from build123d import *

# Parameters (mm, degrees)
SKETCH1_R           = 8
SKETCH1_R_2         = 8.5
BOSS_EXTRUDE1_DEPTH = 35
BOSS_EXTRUDE3_DEPTH = 12
CUT_EXTRUDE1_DEPTH  = 14.407172
SKETCH7_R           = 8.5
BOSS_EXTRUDE4_DEPTH = 15
SKETCH7_3_R         = 5
CUT_EXTRUDE2_DEPTH  = 15
SKETCH7_4_R         = 6.165
CUT_EXTRUDE3_DEPTH  = 1.5
SKETCH7_5_R         = 1.425
CUT_EXTRUDE4_DEPTH  = 8


with BuildPart() as part:
    # Sketch1 → Boss-Extrude1 (new body)
    with BuildSketch(Plane(origin=(0, 0, 0), x_dir=(1, 0, 0), z_dir=(0, 1, 0))):
        with BuildLine():
            ThreePointArc((-50.982546594, 7.568285795), (-54, 0), (-50.982546594, -7.568285795))
            Line((-50.982546594, -7.568285795), (-54, -11))
            Line((-54, -11), (-54, -25.34082208))
            Line((-54, -25.34082208), (-47.34082208, -32))
            Line((-47.34082208, -32), (5, -32))
            Line((5, -32), (15.759494281, -19.407172386))
            ThreePointArc((15.759494281, -19.407172386), (18.621320344, -18.621320344), (19.407172386, -15.759494281))
            ThreePointArc((19.407172386, -15.759494281), (25, 0), (19.407172386, 15.759494281))
            ThreePointArc((19.407172386, 15.759494281), (18.621320344, 18.621320344), (15.759494281, 19.407172386))
            Line((15.759494281, 19.407172386), (5, 32))
            Line((5, 32), (1, 32))
            Line((1, 32), (1, 21.977260976))
            ThreePointArc((1, 21.977260976), (8.243992543, 20.396974946), (14.551632211, 16.5))
            Line((14.551632211, 16.5), (16.5, 16.5))
            Line((16.5, 16.5), (16.5, 14.551632211))
            ThreePointArc((16.5, 14.551632211), (22, 0), (16.5, -14.551632211))
            Line((16.5, -14.551632211), (16.5, -16.5))
            Line((16.5, -16.5), (14.551632211, -16.5))
            ThreePointArc((14.551632211, -16.5), (0, -22), (-14.551632211, -16.5))
            Line((-14.551632211, -16.5), (-16.5, -16.5))
            Line((-16.5, -16.5), (-16.5, -14.551632211))
            ThreePointArc((-16.5, -14.551632211), (-22, 0), (-16.5, 14.551632211))
            Line((-16.5, 14.551632211), (-16.5, 16.5))
            Line((-16.5, 16.5), (-14.551632211, 16.5))
            ThreePointArc((-14.551632211, 16.5), (-8.243992543, 20.396974946), (-1, 21.977260976))
            Line((-1, 21.977260976), (-1, 32))
            Line((-1, 32), (-47.34082208, 32))
            Line((-47.34082208, 32), (-54, 25.34082208))
            Line((-54, 25.34082208), (-54, 11))
            Line((-54, 11), (-50.982546594, 7.568285795))
        make_face()
        with BuildLine():
            ThreePointArc((-48.638105805, -9.445197877), (-47.038026147, -10.232025451), (-45.331844763, -10.75))
            ThreePointArc((-45.331844763, -10.75), (-48.408051309, -11.921222362), (-51, -13.950165565))
            Line((-51, -13.950165565), (-51, -12.131352314))
            Line((-51, -12.131352314), (-48.638105805, -9.445197877))
        make_face(mode=Mode.SUBTRACT)
        with Locations((-43, -21.5)):
            Circle(SKETCH1_R, mode=Mode.SUBTRACT)
        with BuildLine():
            ThreePointArc((-34.95326153, -29), (-32.502649264, -18.212808567), (-40.668155237, -10.75))
            ThreePointArc((-40.668155237, -10.75), (-37.204464997, -9.349426401), (-34.409357086, -6.870287791))
            Line((-34.409357086, -6.870287791), (-24.037452978, -6.870287791))
            ThreePointArc((-24.037452978, -6.870287791), (-11.513133706, -22.191163833), (8.224630177, -23.60837687))
            Line((8.224630177, -23.60837687), (3.617949295, -29))
            Line((3.617949295, -29), (-34.95326153, -29))
        make_face(mode=Mode.SUBTRACT)
        with Locations((-43, 0)):
            Circle(SKETCH1_R_2, mode=Mode.SUBTRACT)
        with BuildLine():
            ThreePointArc((-45.331844763, 10.75), (-47.038026147, 10.232025451), (-48.638105805, 9.445197877))
            Line((-48.638105805, 9.445197877), (-51, 12.131352314))
            Line((-51, 12.131352314), (-51, 13.950165565))
            ThreePointArc((-51, 13.950165565), (-48.408051309, 11.921222362), (-45.331844763, 10.75))
        make_face(mode=Mode.SUBTRACT)
        with BuildLine():
            ThreePointArc((-32.905418056, -4.370287791), (-32, 0), (-32.905418056, 4.370287791))
            Line((-32.905418056, 4.370287791), (-24.615047931, 4.370287791))
            ThreePointArc((-24.615047931, 4.370287791), (-25, 0), (-24.615047931, -4.370287791))
            Line((-24.615047931, -4.370287791), (-32.905418056, -4.370287791))
        make_face(mode=Mode.SUBTRACT)
        with Locations((-43, 21.5)):
            Circle(SKETCH1_R, mode=Mode.SUBTRACT)
        with BuildLine():
            ThreePointArc((-34.409357086, 6.870287791), (-37.204464997, 9.349426401), (-40.668155237, 10.75))
            ThreePointArc((-40.668155237, 10.75), (-32.502649264, 18.212808567), (-34.95326153, 29))
            Line((-34.95326153, 29), (-4, 29))
            Line((-4, 29), (-4, 24.677925359))
            ThreePointArc((-4, 24.677925359), (-16.607308069, 18.68682206), (-24.037452978, 6.870287791))
            Line((-24.037452978, 6.870287791), (-34.409357086, 6.870287791))
        make_face(mode=Mode.SUBTRACT)
        with BuildLine():
            ThreePointArc((8.223751321, 23.608683026), (6.135213434, 24.235493725), (4, 24.677925359))
            Line((4, 24.677925359), (4, 28.552128404))
            Line((4, 28.552128404), (8.223751321, 23.608683026))
        make_face(mode=Mode.SUBTRACT)
    extrude(amount=BOSS_EXTRUDE1_DEPTH)

    # Sketch6 → Boss-Extrude3 (add)
    with BuildSketch(Plane(origin=(0, 23.5, 0), x_dir=(0, 0, -1), z_dir=(0, -1, 0))):
        Polygon((30.717367885, 3.963704263), (22.785433959, 3.963704263), (22.785433959, 10.604126234), align=None)
    extrude(amount=BOSS_EXTRUDE3_DEPTH)

    # Sketch3 → Cut-Extrude1 (cut)
    with BuildSketch(Plane.ZY.offset(-19.407172386)):
        with BuildLine():
            ThreePointArc((-23, 17.5), (-24.171572875, 20.328427125), (-27, 21.5))
            Line((-27, 21.5), (-27, 13.5))
            ThreePointArc((-27, 13.5), (-24.171572875, 14.671572875), (-23, 17.5))
        make_face()
        with BuildLine():
            Line((-27, 13.5), (-27, 21.5))
            ThreePointArc((-27, 21.5), (-31, 17.5), (-27, 13.5))
        make_face()
        with BuildLine():
            Line((-27, 21.5), (-32, 21.5))
            Line((-32, 21.5), (-32, 13.5))
            Line((-32, 13.5), (-27, 13.5))
            ThreePointArc((-27, 13.5), (-31, 17.5), (-27, 21.5))
        make_face()
    extrude(amount=CUT_EXTRUDE1_DEPTH, mode=Mode.SUBTRACT)

    # Sketch7 → Boss-Extrude4 (add)
    with BuildSketch(Plane.XZ):
        with Locations((-43, 0)):
            Circle(SKETCH7_R)
    extrude(amount=-BOSS_EXTRUDE4_DEPTH)

    # Sketch7<3> → Cut-Extrude2 (cut)
    with BuildSketch(Plane.XZ):
        with Locations((-43, 0)):
            Circle(SKETCH7_3_R)
    extrude(amount=-CUT_EXTRUDE2_DEPTH, mode=Mode.SUBTRACT)

    # Sketch7<4> → Cut-Extrude3 (cut)
    with BuildSketch(Plane.XZ):
        with Locations((-43, 0)):
            Circle(SKETCH7_4_R)
    extrude(amount=-CUT_EXTRUDE3_DEPTH, mode=Mode.SUBTRACT)

    # Sketch7<5> → Cut-Extrude4 (cut)
    with BuildSketch(Plane.XZ):
        with Locations((-48.64603005, -5.667657777)):
            Circle(SKETCH7_5_R)
        with Locations((-48.656854249, 5.656854249)):
            Circle(SKETCH7_5_R)
        with Locations((-37.332342223, 5.667678449)):
            Circle(SKETCH7_5_R)
        with Locations((-37.321518023, -5.656833577)):
            Circle(SKETCH7_5_R)
    extrude(amount=-CUT_EXTRUDE4_DEPTH, mode=Mode.SUBTRACT)


solid = part.part
Design review of the part built by this model. Coordinates are the model's own, in mm. A direction names the side the tool comes from. Round coordinates to 2 decimals unless told otherwise and drop trailing zeros. Write each loop counter-clockwise with the first axis right and the second up, starting at its lowest first coordinate (ties: lowest second). Pieces come first, ordered by that corner, then holes.
Item 1: Consider section B-B on z = 0. Give the boundary of the cut face in (x, y) (3 decimals), and give its area (3 significant figures).
Item 2: Consider section A-A on x = -27.5. Give the boundary of the cut face in (y, z).
Item 3: Wall thickness on L1, parallel to Z at x = -43, y = 0.4 (3 decimals); L2, parallel to Z at x = -29, y = 14.5; L3, parallel to X at y = 5, z = 0.5 (3 decimals): over which ranges is each line inside the solid? List them lowest first.
Item 4: For faces 1 (the cylindrical face through (-49.265, 24.86, -5.745)), 2 (the flat face through (-29, 17, -4.37)), 3 (the flat face through (-54, 17, -18)), list the 3-axis set-ups (+Z, -Z, +X, -X, +Y, -Y) from which the entire face can be reached by the end or side of a thin tool; tool diameter is ignored.
Item 5: Consider section D-D on x = -43. Give the boundary of the cut face in (y, z) (3 decimals).
Item 6: Consider section C-C on y = 24.5. Count the separate pieces of the cut face and the enclosed holes in it, and give its area (3 significant figures).
Item 7: For pin 1 Ø1.9 at (y, z) = (3.5, -27) entering from +X; pin 2 Ø4 at (y, z) = (16, -28) entering from +X; pin 3 Ø2 at (y, z) = (21.5, -15.5) entering from +X, all flat-tipped, find the tip position at first contact; note any pin that passes through.
Item 8: Draft analysis for pull direction Y (two halves, no side actions). For faces 4 (the flat face through (1, 17, -27)), 5 (the flat face through (5, 18, -28)), 6 (the flat face through (-49, 8, -6)), state which applies: released by +Y, released by -Y, zero draft, split by the parting line, or undercut.
Check values:
1. outline: (-54, 0) - (-49.165, 0) - (-49.165, 1.5) - (-48, 1.5) - (-48, 15) - (-51.5, 15) - (-51.5, 35) - (-54, 35) - close; (-38, 1.5) - (-36.835, 1.5) - (-36.835, 0) - (-32, 0) - (-32, 35) - (-34.5, 35) - (-34.5, 15) - (-38, 15) - close; (-25, 0) - (-22, 0) - (-22, 35) - (-25, 35) - close; (22, 0) - (25, 0) - (25, 35) - (22, 35) - close
1. area: 487 mm2
2. outline: (0, -32) - (35, -32) - (35, -29) - (0, -29) - close; (0, -6.87) - (35, -6.87) - (35, -4.37) - (0, -4.37) - close; (0, 4.37) - (35, 4.37) - (35, 6.87) - (0, 6.87) - close; (0, 29) - (35, 29) - (35, 32) - (0, 32) - close
3. L1: z = -32 to -29.5, -13.5 to -6.165, 6.165 to 13.5, 29.5 to 32
3. L2: z = -32 to -29, -6.87 to -4.37, 4.37 to 6.87, 29 to 32
3. L3: x = -53.989 to -47.975, -38.025 to -32.011, -24.995 to -21.994, 21.994 to 24.995
4. face 1: +Y
4. face 2: +Y, -Y
4. face 3: +Z, -Z, -X, +Y, -Y
5. outline: (0, -32) - (35, -32) - (35, -29.5) - (0, -29.5) - close; (0, -13.5) - (35, -13.5) - (35, -8.5) - (15, -8.5) - (15, -5) - (1.5, -5) - (1.5, -6.165) - (0, -6.165) - close; (0, 6.165) - (1.5, 6.165) - (1.5, 5) - (15, 5) - (15, 8.5) - (35, 8.5) - (35, 13.5) - (0, 13.5) - close; (0, 29.5) - (35, 29.5) - (35, 32) - (0, 32) - close
6. separate pieces: 1
6. enclosed holes: 9
6. area: 1,370 mm2
7. pin 1: stops at x = 10.08
7. pin 2: stops at x = 5
7. pin 3: stops at x = 20.37
8. face 4: zero draft
8. face 5: undercut
8. face 6: released by -Y
